from build123d import *

# Parameters (mm, degrees)
SKETCH1_R           = 17.5
SKETCH1_R_2         = 10
BOSS_EXTRUDE1_DEPTH = 20
SKETCH2_R           = 15
SKETCH2_R_2         = 10
BOSS_EXTRUDE2_DEPTH = 50


with BuildPart() as part:
    # Sketch1 → Boss-Extrude1 (new body)
    with BuildSketch(Plane.XY):
        with BuildLine():
            Line((0, 138), (0, 0))
            Line((0, 0), (522.5, 0))
            Line((522.5, 0), (522.5, 60))
            Line((522.5, 60), (374.649400312, 86.070049839))
            Line((374.649400312, 86.070049839), (244.94, 310.733321399))
            ThreePointArc((244.94, 310.733321399), (200.912248971, 330.848790378), (153, 337.740187298))
            Line((153, 337.740187298), (153, 281.918848091))
            Line((153, 281.918848091), (4.984782256, 149.166710059))
            ThreePointArc((4.984782256, 149.166710059), (1.302769146, 144.114398329), (0, 138))
        make_face()
        with Locations((153, 167.740187298)):
            Circle(SKETCH1_R, mode=Mode.SUBTRACT)
        with Locations((15, 138)):
            Circle(SKETCH1_R_2, mode=Mode.SUBTRACT)
    extrude(amount=BOSS_EXTRUDE1_DEPTH)

    # Sketch2 → Boss-Extrude2 (add)
    with BuildSketch(Plane.XY.offset(20)):
        with Locations((15, 138)):
            Circle(SKETCH2_R)
        with Locations((15, 138)):
            Circle(SKETCH2_R_2, mode=Mode.SUBTRACT)
    extrude(amount=BOSS_EXTRUDE2_DEPTH)


solid = part.part
CAD build for the part. Positions are in the model's coordinates, mm. A direction names the side the tool comes from. Round coordinates to 2 decimals unless told otherwise and drop trailing zeros. Write each loop counter-clockwise with the first axis right and the second up, starting at its lowest first coordinate (ties: lowest second). Pieces come first, ordered by that corner, then holes. Notation, with made-up numbers: M 5.5,-29.5 L 11.5,-29.5 A35 cw 11.5,7.5 Z; hole C 44.25,40 d6. An arc over 180 degrees is marked long. Use a Markdown table: item, result. Add a question column.
1. Flat gauge pins, fed straight in: P1, Ø1, axis at x = 396, z = 13, coming from the +Y side; P2, Ø10, axis at x = 287, y = 188.5, coming from the +Z side; P3, Ø6, axis at y = 308, z = 10.5, coming from the -X side. Where does each tip first touch, or does it go through?
2. Pull direction Y, two halves, no side cores. Call faces 1 (the face through (200, 134, 0)), 2 (the face through (80.028, 216.472, 9.86)), 3 (the face through (20.38, 146.43, 34.51)): released by +Y, released by -Y, zero draft, split by the parting line, or undercut.
3. Slice it at B-B on z = 54. Give the cut face in (x, y).
4. Slice it at D-D on x = 199.5. Give the cut face in (y, z).
5. 3-axis set-ups, long thin cutter, end or side, ignore diameter. For faces 4 (the face through (153, 310, 10)), 5 (the face through (25, 135, 70)): which of +Z, -Z, +X, -X, +Y, -Y reach the whole face in a straight line?
6. Drill centre lines: probe 1 along Y at (x, z) = (15, 55); probe 2 along Z at (x, y) = (280, 166); probe 3 along X at (y, z) = (123, 10). Where is each one in solid material? Low to high.
7. Slice it at C-C on y = 108. Give the cut face in (x, z), then the cut area to 3 significant figures.
8. Slice it at A-A on x = 15. Give the cut face in (y, z).
Reply:
| question | item | result |
|---|---|---|
| 1 | P1 | stops at y = 82.39 |
| 1 | P2 | stops at z = 20 |
| 1 | P3 | stops at x = 153 |
| 2 | face 1 | zero draft |
| 2 | face 2 | released by +Y |
| 2 | face 3 | undercut |
| 3 | outline | C 15,138 d30; hole C 15,138 d20 |
| 4 | outline | M 0,0 L 331.26,0 L 331.26,20 L 0,20 Z |
| 5 | face 4 | +Z, -Z, -X, +Y |
| 5 | face 5 | +Z, +X, -X, +Y, -Y |
| 6 | probe 1 | y = 123 to 128, 148 to 153 |
| 6 | probe 2 | z = 0 to 20 |
| 6 | probe 3 | x = 0 to 353.33 |
| 7 | outline | M 0,0 L 361.99,0 L 361.99,20 L 0,20 Z |
| 7 | area | 7,240 mm^2 |
| 8 | outline | M 0,0 L 128,0 L 128,70 L 123,70 L 123,20 L 0,20 Z; M 148,0 L 158.15,0 L 158.15,20 L 153,20 L 153,70 L 148,70 Z |
